For this review, use the dimensioned drawing (mm, ordinates from the lowest corner) and the shaded views. A direction names the side the tool comes from. Round coordinates to 2 decimals unless told otherwise and drop trailing zeros. Write each loop counter-clockwise with the first axis right and the second up, starting at its lowest first coordinate (ties: lowest second). Pieces come first, ordered by that corner, then holes. Notation, with made-up numbers: M 80,79 L 116,79 A23 cw 116,113 Z; hole C 40.5,-6 d10. An arc over 180 degrees is marked long. Use one line per item in the form item = value. Start each with the question number.
Item 1: Add section A-A (y = 32.7). State the section outline as (x, z) points.
Item 2: For line 1 (Y direction, x = 35.88, z = 1.85) (3 decimals); line 2 (X direction, y = 8.5, z = 6.25); line 3 (Y direction, x = 6, z = 5.5), list the stretches that pass through material, from the lowest coordinate up. Write a range as [from, to].
Item 3: For the marked faces 4 and 5, list the 3-axis set-ups (+Z, -Z, +X, -X, +Y, -Y) from which the entire face can be reached by the end or side of a thin tool; tool diameter is ignored.
Item 4: Draft analysis for pull direction X (two halves, no side actions). For the marked faces 1, 2 and 3, state which applies: released by +X, released by -X, zero draft, split by the parting line, or undercut.
Item 5: Add section B-B (z = 8.75). State the section outline as (x, y) points.
Item 6: For P1, Ø3, axis at x = 32, y = 33, coming from the +Z side; P2, Ø1.3, axis at x = 35.5, y = 36, coming from the -Z side, all flat-tipped, find the tip position at first contact; note any pin that passes through.
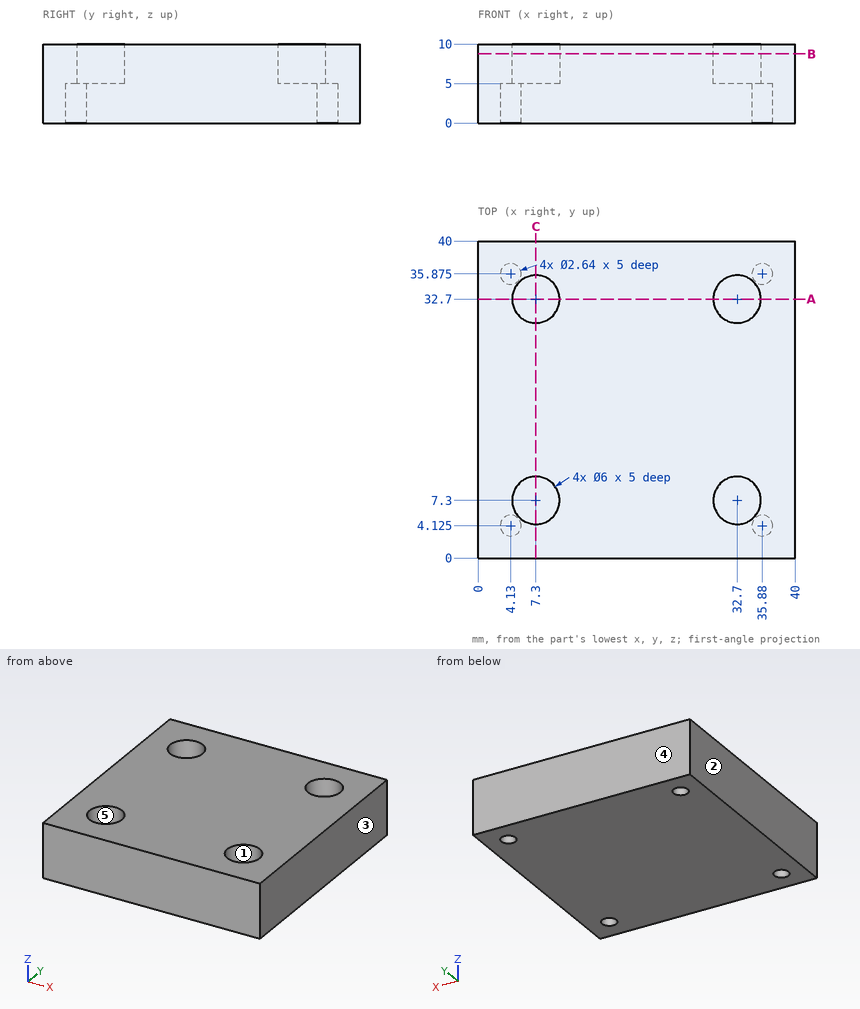
Calculated:
q1.outline = M 0,0 L 40,0 L 40,10 L 35.7,10 L 35.7,5 L 29.7,5 L 29.7,10 L 10.3,10 L 10.3,5 L 4.3,5 L 4.3,10 L 0,10 Z
q2.line_1 = [0, 2.805], [5.445, 34.555], [37.195, 40]
q2.line_2 = [0, 4.55], [10.05, 29.95], [35.45, 40]
q2.line_3 = [0, 4.6], [10, 30], [35.4, 40]
q3.face_4 = +Z, -Z, +X, -X, +Y
q3.face_5 = +Z
q4.face_1 = undercut
q4.face_2 = released by -X
q4.face_3 = released by +X
q5.outline = M 0,0 L 40,0 L 40,40 L 0,40 Z; hole C 7.3,7.3 d6; hole C 7.3,32.7 d6; hole C 32.7,7.3 d6; hole C 32.7,32.7 d6
q6.P1 = 5
q6.P2 = 5
